```python
from build123d import *

# Parameters (mm, degrees)
SKETCH1_W               = 700
SKETCH1_H               = 500
BOSS_EXTRUDE1_DEPTH     = 500
CUT_EXTRUDE1_DEPTH      = 1
CUT_EXTRUDE1_DEPTH_BACK = 500
CUT_EXTRUDE2_DEPTH      = 1
CUT_EXTRUDE2_DEPTH_BACK = 350


with BuildPart() as part:
    # Sketch1 → Boss-Extrude1 (new body)
    with BuildSketch(Plane(origin=(0, 0, 0), x_dir=(1, 0, 0), z_dir=(0, 1, 0))):
        with Locations((350, 250)):
            Rectangle(SKETCH1_W, SKETCH1_H)
    extrude(amount=BOSS_EXTRUDE1_DEPTH)

    # Sketch3 → Cut-Extrude1 (cut, two sides)
    with BuildSketch(Plane(origin=(700, 0, 0), x_dir=(0, 0, -1), z_dir=(1, 0, 0))) as cut_extrude1_sk:
        Polygon((0, 100), (250, 500), (0, 500), align=None)
    extrude(amount=CUT_EXTRUDE1_DEPTH, mode=Mode.SUBTRACT)
    extrude(cut_extrude1_sk.sketch, amount=-CUT_EXTRUDE1_DEPTH_BACK, mode=Mode.SUBTRACT)

    # Sketch3_3 → Cut-Extrude2 (cut, two sides)
    with BuildSketch(Plane(origin=(700, 0, 0), x_dir=(0, 0, -1), z_dir=(1, 0, 0))) as cut_extrude2_sk:
        Polygon((500, 500), (250, 500), (500, 280), align=None)
    extrude(amount=CUT_EXTRUDE2_DEPTH, mode=Mode.SUBTRACT)
    extrude(cut_extrude2_sk.sketch, amount=-CUT_EXTRUDE2_DEPTH_BACK, mode=Mode.SUBTRACT)


solid = part.part
```
Geometry check sheet. Reference: the model listing, model coordinates, mm. A direction names the side the tool comes from. Coordinates: 2 decimals unless noted, no trailing zeros. Loops run counter-clockwise (first coordinate to the right, second up) from the corner with the lowest first, then second, coordinate; pieces in that order, holes last.
Item 1: Thickness scan on line 1 (X direction, y = 410.5, z = -443.5); line 2 (X direction, y = 363, z = -38); line 3 (Y direction, x = 507, z = -303.5). Record the ranges inside material, lowest first.
Item 2: Sectioned sample at B-B, the plane y = 368. Record the boundary of the cut face in (x, z), then the cut area to 3 significant figures.
Item 3: Go/stop test with flat-tipped pins: pin 1 Ø3 at (x, y) = (505.5, 287.5) entering from +Z; pin 2 Ø6 at (y, z) = (401.5, -376.5) entering from +X; pin 3 Ø6 at (x, y) = (332.5, 231) entering from +Z. Record where each tip stops, or that it passes through.
Item 4: Access from +Z, -Z, +X, -X, +Y, -Y to the whole of each face (thin tool, end or side, straight path). Record for faces 1 (the face through (350, 440, -429)), 2 (the face through (453.5, 297.2, -123.25)), 3 (the face through (267, 191, -500)).
Item 5: Sectioned sample at D-D, the plane z = -134. Record the boundary of the cut face in (x, y), then the cut area to 3 significant figures.
Item 6: Sectioned sample at A-A, the plane z = -442.5. Record the boundary of the cut face in (x, y).
Item 7: Sectioned sample at C-C, the plane x = 213. Record the boundary of the cut face in (y, z).
Check result:
1. line 1: x = 0 to 350
1. line 2: x = 0 to 200
1. line 3: y = 0 to 452.92
2. outline: (0, -500) - (350, -500) - (350, -400) - (700, -400) - (700, -167.5) - (200, -167.5) - (200, 0) - (0, 0) - close
2. area: 231,000 mm2
3. pin 1: stops at z = -116.25
3. pin 2: stops at x = 350
3. pin 3: stops at z = -80
4. face 1: -Z, +X, +Y
4. face 2: +Z, +X, +Y
4. face 3: -Z, +X, -X, +Y, -Y
5. outline: (0, 0) - (700, 0) - (700, 314.4) - (200, 314.4) - (200, 500) - (0, 500) - close
5. area: 257,000 mm2
6. outline: (0, 0) - (700, 0) - (700, 330.6) - (350, 330.6) - (350, 500) - (0, 500) - close
7. outline: (0, -500) - (500, -500) - (500, -250) - (100, 0) - (0, 0) - close
